Design review of the part built by this model. Coordinates are the model's own, in mm. Face numbers are marked on the shaded views. Coordinates: 2 decimals unless noted, no trailing zeros. Loops run counter-clockwise (first coordinate to the right, second up) from the corner with the lowest first, then second, coordinate; pieces in that order, holes last.
from build123d import *

# Parameters (mm, degrees)
SKETCH_1_R          = 30
SKETCH_1_R_2        = 12.5
EXTRUDE_1_DEPTH     = 4
SKETCH_2_R          = 1.6
CUT_EXTRUDE_1_DEPTH = 4
SKETCH_3_R          = 1.4
CUT_EXTRUDE_2_DEPTH = 10


with BuildPart() as part:
    # 草图1 → 凸台-拉伸1 (new body)
    with BuildSketch(Plane(origin=(0, 0, 0), x_dir=(1, 0, 0), z_dir=(0, 1, 0))):
        with Locations(Location((0, 0, 0), (0, 0, 270))):
            Circle(SKETCH_1_R)
        with Locations(Location((0, 0, 0), (0, 0, 270))):
            Circle(SKETCH_1_R_2, mode=Mode.SUBTRACT)
    extrude(amount=EXTRUDE_1_DEPTH)

    # 草图2 → 切除-拉伸1 (cut)
    with BuildSketch(Plane(origin=(0, 4, 0), x_dir=(1, 0, 0), z_dir=(0, 1, 0))):
        with Locations(Location((11, 11, 0), (0, 0, 270))):
            Circle(SKETCH_2_R)
        with Locations(Location((11, -11, 0), (0, 0, 270))):
            Circle(SKETCH_2_R)
        with Locations(Location((-11, -11, 0), (0, 0, 270))):
            Circle(SKETCH_2_R)
        with Locations(Location((-11, 11, 0), (0, 0, 270))):
            Circle(SKETCH_2_R)
    extrude(amount=-CUT_EXTRUDE_1_DEPTH, mode=Mode.SUBTRACT)

    # 草图3 → 切除-拉伸2 (cut)
    with BuildSketch(Plane(origin=(0, 4, 0), x_dir=(1, 0, 0), z_dir=(0, 1, 0))):
        with Locations(Location((23.5, 0, 0), (0, 0, 270))):
            Circle(SKETCH_3_R)
        with Locations(Location((-11.75, 20.351596989, 0), (0, 0, 270))):
            Circle(SKETCH_3_R)
        with Locations(Location((-11.75, -20.351596989, 0), (0, 0, 270))):
            Circle(SKETCH_3_R)
    extrude(amount=-CUT_EXTRUDE_2_DEPTH, mode=Mode.SUBTRACT)


solid = part.part
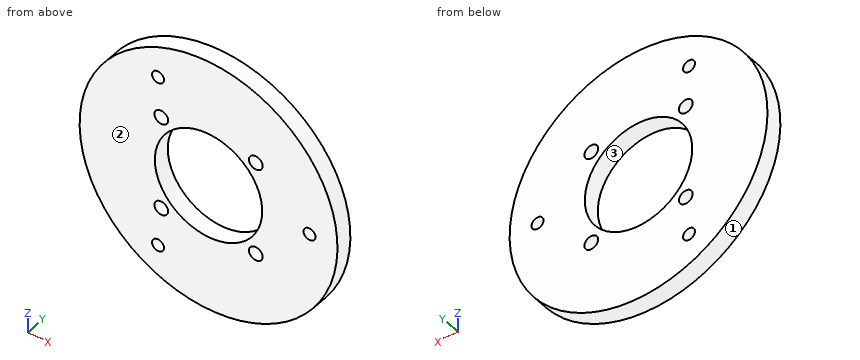
Q1. Take a section at A-A, the plane x = 0. Write out the cut boundary in (y, z), then the cut area to 3 significant figures.
Q2. Take a section at C-C, the plane y = 0.6. Give the number of separate pieces and of enclosed holes in the cut face, then the cut area to 3 significant figures.
Q3. Take a section at D-D, the plane x = -11.75. Write out the cut boundary in (y, z).
Q4. For line 1 (X direction, y = 2.1, z = 0); line 2 (X direction, y = 1.4, z = -11); line 3 (X direction, y = 2.15, z = -6), list the stretches that pass through material, from the lowest coordinate up.
Q5. Clearance check with flat-ended pins moving along their axes: pin 1 Ø2 at (y, z) = (3, -9.5) entering from +X; pin 2 Ø2 at (y, z) = (3.5, 23.5) entering from -X; pin 3 Ø1.5 at (x, y) = (18.5, 3) entering from -Z. State where each tip first meets the part, or that it passes through.
Q6. Take a section at B-B, the plane z = -5.5. Write out the cut boundary in (x, y).
Q7. The part is to be moulded in two halves that separate along X. For the marked faces 1, 2 and 3, say which applies: pulls with the +X half, pulls with the -X half, needs draft (parallel to the pull), parting line crosses it, or undercut.
Entries:
1. outline: (0, -30) - (4, -30) - (4, -12.5) - (0, -12.5) - close; (0, 12.5) - (4, 12.5) - (4, 30) - (0, 30) - close
1. area: 140 mm2
2. separate pieces: 1
2. enclosed holes: 8
2. area: 2,290 mm2
3. outline: (0, -27.6) - (4, -27.6) - (4, -21.75) - (0, -21.75) - close; (0, -18.95) - (4, -18.95) - (4, -12.41) - (0, -12.41) - close; (0, -9.59) - (4, -9.59) - (4, -4.26) - (0, -4.26) - close; (0, 4.26) - (4, 4.26) - (4, 9.59) - (0, 9.59) - close; (0, 12.41) - (4, 12.41) - (4, 18.95) - (0, 18.95) - close; (0, 21.75) - (4, 21.75) - (4, 27.6) - (0, 27.6) - close
4. line 1: x = -30 to -12.5, 12.5 to 22.1, 24.9 to 30
4. line 2: x = -27.91 to -12.6, -9.4 to -5.94, 5.94 to 9.4, 12.6 to 27.91
4. line 3: x = -29.39 to -10.97, 10.97 to 29.39
5. pin 1: stops at x = 28.77
5. pin 2: stops at x = -19.84
5. pin 3: stops at z = -24.19
6. outline: (-29.49, 0) - (-11.22, 0) - (-11.22, 4) - (-29.49, 4) - close; (11.22, 0) - (29.49, 0) - (29.49, 4) - (11.22, 4) - close
7. face 1: parting line crosses it
7. face 2: needs draft
7. face 3: undercut
